Drawing for the job (mm, zero at the part's lowest x, y, z). A direction names the side the tool comes from. Round coordinates to 2 decimals unless told otherwise and drop trailing zeros. Write each loop counter-clockwise with the first axis right and the second up, starting at its lowest first coordinate (ties: lowest second). Pieces come first, ordered by that corner, then holes.
Item 1: Wall check: probe 1 along Z at (x, y) = (0.6, 3.5); probe 2 along Y at (x, z) = (2.7, 5) (1 decimal); probe 3 along X at (y, z) = (3.25, 10). Give the ranges that are in metal, low to high.
Item 2: Drop flat-ended pins along their axis: pin 1 Ø2 at (x, z) = (4.5, 8.5) entering from -Y; pin 2 Ø1 at (x, z) = (3, 13.5) entering from -Y (1 decimal). Give the stop position or say it passes through.
Item 3: Band-saw the part on A-A, the plane z = 1.75. Write the cut outline in (x, y), then the cut area to 3 significant figures.
Item 4: 3-axis set-ups, long thin cutter, end or side, ignore diameter. For the marked faces 1 and 2: which of +Z, -Z, +X, -X, +Y, -Y reach the whole face in a straight line?
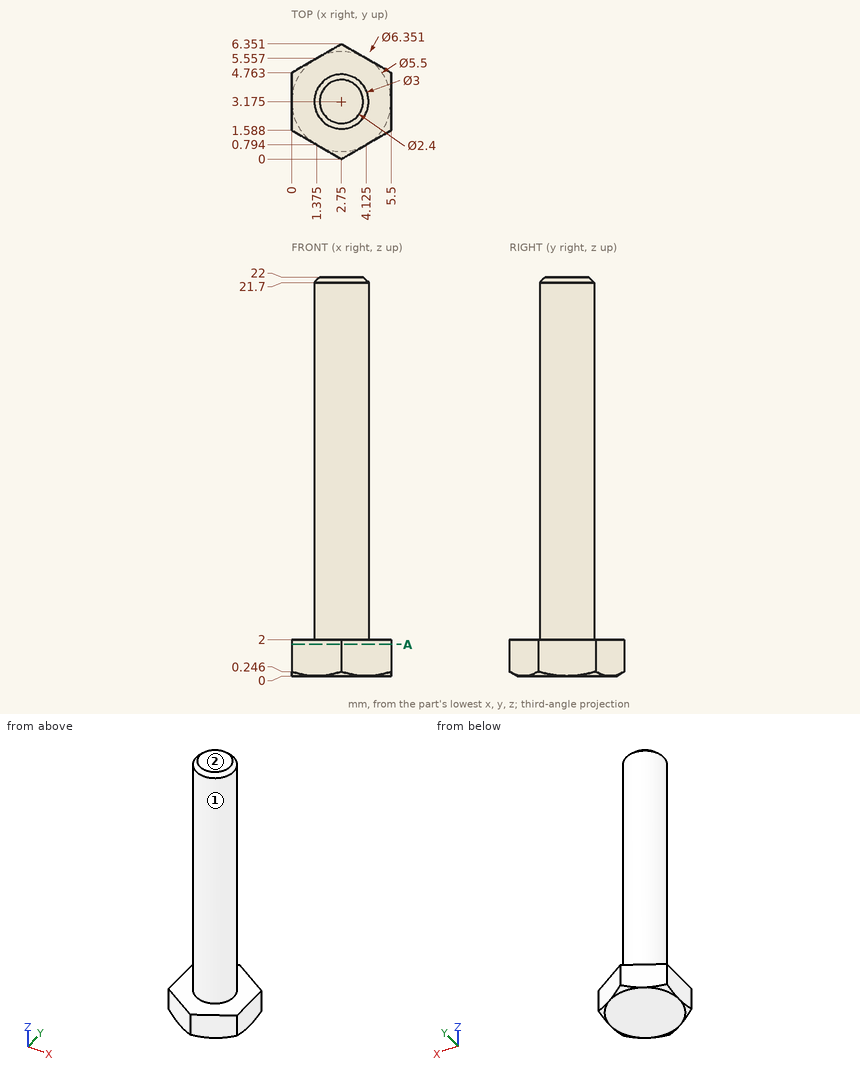
Results:
1. probe 1: z = 0 to 2
1. probe 2: y = 1.7 to 4.7
1. probe 3: x = 1.25 to 4.25
2. pin 1: stops at y = 1.88
2. pin 2: stops at y = 1.7
3. outline: (0, 1.59) - (2.75, 0) - (5.5, 1.59) - (5.5, 4.76) - (2.75, 6.35) - (0, 4.76) - close
3. area: 26.2 mm2
4. face 1: +Z
4. face 2: +Z, +X, -X, +Y, -Y
